Verification items for the finished model (mm, model axes). Face numbers are marked on the shaded views. A direction names the side the tool comes from. Coordinates: 2 decimals unless noted, no trailing zeros. Order: outer loops, then holes, each group sorted by start corner. A loop starts at its lowest first (then second) coordinate and runs counter-clockwise, first axis right, second up. Notation, with made-up numbers: M -3.75,65.5 L 22.25,65.5 A30 cw 22.25,104.5 Z; hole C 37,47 d8. An arc over 180 degrees is marked long. Return JSON: item names as keys, results as strings. Group by question number.
1. Section check B-B, the plane y = -40. Record the cut outline in (x, z) (3 decimals), plus the area to 3 significant figures.
2. Set-up check for the marked faces 4, 5 and 6: record each of +Z, -Z, +X, -X, +Y, -Y from which the full face is reachable in a straight line by a thin tool's end or side.
3. Mould release check, pull along Y, two halves, no side actions. Record for the marked faces 1, 2 and 3: +Y half, -Y half, draft (parallel to the pull), parting line (faces both ways), or undercut.
4. Section check A-A, the plane z = 24. Record the cut outline in (x, y), plus the area to 3 significant figures.
5. Material ranges on line 1 along Y through (x, z) = (1.5, 15.5); line 2 along Y through (x, z) = (-12, 24); line 3 along Z through (x, y) = (24.5, -46), recorded low to high.
6. Section check C-C, the plane x = -32. Record the cut outline in (y, z), plus the area to 3 significant figures.
7. Gauge pin test, flat ends, axial feed: pin 1 (24 mm diameter, centred on x = -13, y = -11, fed in from +Z); pin 2 (10 mm diameter, centred on y = -37, z = 2, fed in from -X); pin 3 (3 mm diameter, centred on y = -51.5, z = 21, fed in from +X); pin 4 (5.5 mm diameter, centred on x = -5.9, z = 12.86, fed in from -Y). Record the tip position at first contact, or that the pin passes through.
```python
from build123d import *

# Parameters (mm, degrees)
F1_DEPTH  = 25.4
F3_D      = 25.4
F3_DEPTH  = 12.7
F3_TIP    = 7.6309298617
F5_DEPTH  = 6.35
F7_D      = 6.35
F7_DEPTH  = 254
F7_TIP    = 1.9077324654
F9_DEPTH  = 6.35
F11_DEPTH = 6.35


with BuildPart() as f1:
    # F0 (on Top) → F1 (new body)
    with BuildSketch(Plane.XY):
        with BuildLine():
            Line((4.4096680358, 46.9340346754), (-17.3225291073, 46.9340346754))
            Line((-17.3225291073, 46.9340346754), (-37.1629750587, 31.0344995595))
            ThreePointArc((-37.1629750587, 31.0344995595), (-46.5261500129, 13.9975710547), (-41.0999868401, -4.6701211252))
            Line((-41.0999868401, -4.6701211252), (-25.2276921751, -24.4765747183))
            Line((-25.2276921751, -24.4765747183), (-26.0085705919, -24.951683338))
            ThreePointArc((-26.0085705919, -24.951683338), (-38.1533474778, -45.0139671836), (-28.6899548002, -66.4717172459))
            Line((-28.6899548002, -66.4717172459), (-17.3225291073, -75.5812302232))
            Line((-17.3225291073, -75.5812302232), (4.4096680358, -75.5812302232))
            Line((4.4096680358, -75.5812302232), (15.7770905265, -66.4717187425))
            ThreePointArc((15.7770905265, -66.4717187425), (25.2404819789, -45.0139682034), (13.0957040513, -24.9516850564))
            Line((13.0957040513, -24.9516850564), (12.3148227185, -24.4765747183))
            Line((12.3148227185, -24.4765747183), (28.1871199764, -4.6701202151))
            ThreePointArc((28.1871199764, -4.6701202151), (33.6132842187, 13.9975716539), (24.2501102406, 31.0345006951))
            Line((24.2501102406, 31.0345006951), (4.4096680358, 46.9340346754))
        make_face()
    extrude(amount=F1_DEPTH)

    # F3
    with Locations(Plane.XY.offset(25.4)):
        with Locations((-6.0439212248, 18.131762743), (-9.2097837478, -25.3269076347)):
            Hole(F3_D / 2, depth=F3_DEPTH)
            with Locations((0, 0, -(F3_DEPTH + F3_TIP / 2))):  # 118° drill point
                Cone(0, F3_D / 2, F3_TIP, mode=Mode.SUBTRACT)

    # F4 (on face) → F5 (join)
    with BuildSketch(Plane.XY.offset(25.4)):
        Polygon((-11.431774831, -59.9473722219), (-1.8083986281, -54.0896646738), (-4.4056227723, -43.1271588469), (-15.6341717727, -42.2096651921), (-19.9765725551, -52.6051287559), align=None)
    extrude(amount=F5_DEPTH)

    # F7
    with Locations(Plane.XZ.offset(75.5812302232)):
        with Locations((-5.8986586519, 12.8560494632)):
            Hole(F7_D / 2, depth=F7_DEPTH)
            with Locations((0, 0, -(F7_DEPTH + F7_TIP / 2))):  # 118° drill point
                Cone(0, F7_D / 2, F7_TIP, mode=Mode.SUBTRACT)

    # F8 (on face) → F9 (join)
    with BuildSketch(Plane(origin=(0, 0, 0), x_dir=(1, 0, 0), z_dir=(0, 0, -1))):
        Polygon((-7.4111339636, -24.9558594078), (0, -25.5608521402), (0, -16.788488254), (8.3186198026, -16.788488254), (8.3663046534, -11.2136853721), (0, -11.1421230232), (0, 0), (-7.4111339636, 0), (-7.4111339636, -11.1421230232), (-14.6710202098, -11.1421230232), (-14.6710202098, -16.788488254), (-7.4111339636, -16.788488254), align=None)
    extrude(amount=F9_DEPTH)

    # F10 (on face) → F11 (join)
    with BuildSketch(Plane(origin=(0, 0, 0), x_dir=(1, 0, 0), z_dir=(0, 0, -1))):
        Polygon((-14.6710202098, 12.5811770558), (10.4360869154, 11.0410777852), (10.4360869154, 21.3259179145), (-14.6710202098, 21.3259179145), align=None)
    extrude(amount=F11_DEPTH)


solid = f1.part
```
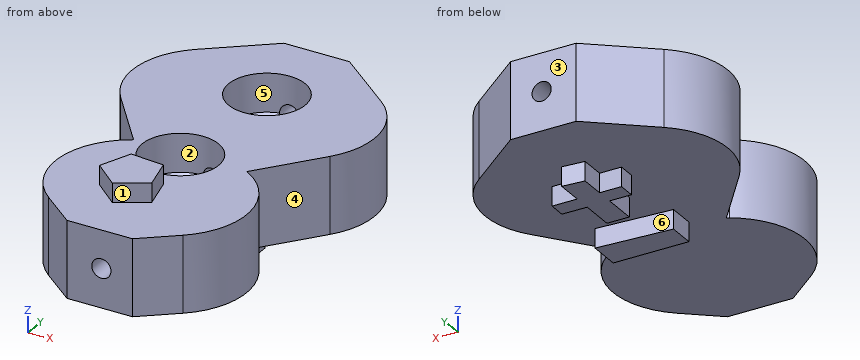
Answers follow:
{
 "1": {"outline": "M -37.32,0 L 24.407,0 L 24.407,25.4 L -37.32,25.4 Z; hole C -5.899,12.856 d6.35", "area": "1,540 mm^2"},
 "2": {"face 4": "+Z, -Z, +X", "face 5": "+Z", "face 6": "-Z, -X"},
 "3": {"face 1": "-Y half", "face 2": "undercut", "face 3": "+Y half"},
 "4": {"outline": "M -41.1,-4.67 L -25.23,-24.48 L -26.01,-24.95 A25.4 ccw -28.69,-66.47 L -17.32,-75.58 L 4.41,-75.58 L 15.78,-66.47 A25.4 ccw 13.1,-24.95 L 12.31,-24.48 L 28.19,-4.67 A25.4 ccw 24.25,31.03 L 4.41,46.93 L -17.32,46.93 L -37.16,31.03 A25.4 ccw Z; hole C -9.21,-25.33 d25.4; hole C -6.04,18.13 d25.4", "area": "6,090 mm^2"},
 "5": {"line 1": "-75.58 to -32.15, -18.5 to 7.92, 28.35 to 46.93", "line 2": "-75.58 to -37.72, -12.94 to 6.92, 29.35 to 46.93", "line 3": "0 to 25.4"},
 "6": {"outline": "M -63.29,0 L -30.01,0 L -30.01,25.4 L -63.29,25.4 Z; M -16.03,0 L 35.17,0 L 35.17,25.4 L -16.03,25.4 Z", "area": "2,150 mm^2"},
 "7": {"pin 1": "z = 25.4", "pin 2": "x = -37.78", "pin 3": "x = 25.07", "pin 4": "through"}
}
